Source: CAD feature listing. Evaluate the final solid. Frame: model axes, mm. Face numbers are marked on the shaded views. A direction names the side the tool comes from. Give positions to 0.01 mm unless a question says otherwise; leave off trailing zeros. Order: outer loops, then holes, each group sorted by start corner. A loop starts at its lowest first (then second) coordinate and runs counter-clockwise, first axis right, second up. Notation, with made-up numbers: (-4.75, -4.75) -> (21.25, -4.75) arc R29 ccw to (21.25, 32.25) -> close; hole circle Ø8 at (33.5, 10). An arc over 180 degrees is marked (long way). Answer in a Markdown table with one row per item.
Autodesk Inventor part; units mm, degrees
ref_plane "YZ Plane" through (0, 0, 0) normal (1, 0, 0) x (0, 1, 0)
ref_plane "XZ Plane" through (0, 0, 0) normal (0, 1, 0) x (-1, 0, 0)
ref_plane "XY Plane" through (0, 0, 0) normal (0, 0, 1) x (1, 0, 0)
sketch "Sketch1" plane through (0, 0, 0) normal (0, 0, 1) x (1, 0, 0)
  line L0 (0, 34.8483) -> (20, 34.8483)
  line L1 (20, 34.8483) -> (20, 29.9983)
  line L2 (0, 34.8483) -> (0, 0)
  line L3 (20, 29.9983) -> (5, 29.9983)
  line L4 (5, 29.9983) -> (5, 7.1983)
  line L5 (5, 7.1983) -> (20, 7.1983)
  line L6 (20, 7.1983) -> (20, 2.3483)
  line L7 (20, 2.3483) -> (5, 2.3483)
  line L8 (0, 0) -> (0, -15.1517)
  line L9 (5, -15.1517) -> (5, 2.3483)
  line L10 (5, -15.1517) -> (5, -22.2152)
  arc A0 (0, -15.1517) -> (5, -22.2152) centre (9.8436, -13.4852) ccw
  dimension "d14" = 20
  dimension "d15" = 4.85
  dimension "d17" = 4.85
  dimension "d18" = 22.8
  dimension "d19" = 20
  dimension "d20" = 5
  dimension "d22" = 9.9837
  dimension "d23" = 90
  dimension "d24" = 29.9983
  dimension "d25" = 10.1564
  dimension "d26" = 43.4835
  dimension "d27" = 45.15
extrude "Extrusion1" add sketch "Sketch1" against normal blind 10
sketch "Sketch2" plane through (20, 29.9983, 0) normal (1, 0, 0) x (0, 0, -1)
  line L0 (0, 0) -> (10, 0)
  line L1 (2, 0) -> (2, 4.85)
  line L2 (0, 4.85) -> (10, 4.85)
  line L3 (2, 4.85) -> (10, 4.85)
  line L4 (10, 4.85) -> (10, 0)
  line L5 (10, -45.15) -> (10, 4.85)
  line L6 (0, 0) -> (0, 4.85)
  line L7 (0, 0) -> (10, 0)
  line L8 (2, 0) -> (10, 0)
  line L9 (10, -22.8) -> (10, -27.65)
  line L10 (2, -27.65) -> (2, -22.8)
  line L11 (2, -22.8) -> (10, -22.8)
  line L12 (10, -22.8) -> (10, -27.65)
  line L13 (2, -27.65) -> (10, -27.65)
  point P0 (0, -29.9983)
  point P1 (10, -11.4)
  dimension "d30" = 2
  dimension "d33" = 11.4
  dimension "d36" = 27.65
extrude "Extrusion2" cut sketch "Sketch2" against normal blind 15 contours L5 L13 L10 L11 | L1 L2 L4 L0
fillet "Fillet1" radius 1 1 edges at (5, -22.2152, -5)
sketch "Sketch3" plane through (0, 0, 0) normal (0, 0, 1) x (1, 0, 0)
  line L0 (20, 34.8483) -> (0, 34.8483)
  line L1 (5, 7.1983) -> (5, 29.9983)
  circle A0 centre (11.05, 32.4233) radius 1.1
  circle A1 centre (11.05, 4.7733) radius 1.1
  point P0 (0, 0)
  dimension "d42" = 2.425
  dimension "d43" = 6.05
  dimension "d44" = 1.1
  dimension "d47" = 27.65
extrude "Extrusion3" cut sketch "Sketch3" against normal blind 15
properties part number "first joint"
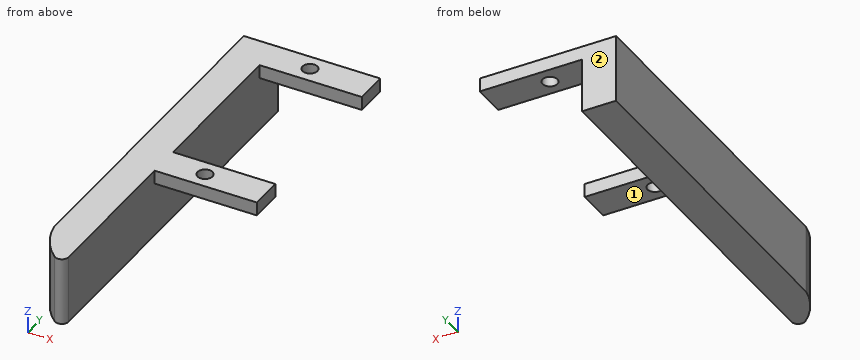
(1) First-contact query: pin 1 Ø5.5 at (x, y) = (9.5, 4.5) entering from -Z; pin 2 Ø1.6 at (x, z) = (15, -1) entering from -Y; pin 3 Ø3 at (x, z) = (12.5, -5) entering from -Y. Flat tips, straight axial feed; report the tip coordinate or a pass-through.
A:
| item | result |
|---|---|
| pin 1 | stops at z = -2 |
| pin 2 | stops at y = 2.35 |
| pin 3 | passes through |
(2) Section query D-D (y = -13). Return the cut outline in (x, z).
A:
| item | result |
|---|---|
| outline | (0, -10) -> (5, -10) -> (5, 0) -> (0, 0) -> close |
(3) Section query C-C (z = -1.5). Return the cut outline in (x, y), plus the area to 3 significant figures.
A:
| item | result |
|---|---|
| outline | (0, -15.15) arc R9.98 ccw to (3.35, -21.07) arc R1 ccw to (5, -20.31) -> (5, 2.35) -> (20, 2.35) -> (20, 7.2) -> (5, 7.2) -> (5, 30) -> (20, 30) -> (20, 34.85) -> (0, 34.85) -> close; hole circle Ø2.2 at (11.05, 4.77); hole circle Ø2.2 at (11.05, 32.42) |
| area | 410 mm^2 |
(4) Ray query, probe 1 along Y at (x, z) = (11.05, -0.65); probe 2 along Y at (x, z) = (17.75, -1); probe 3 along Z at (x, y) = (19, 6). Return the intervals inside material, ascending.
A:
| item | result |
|---|---|
| probe 1 | y = 2.35 to 3.67, 5.87 to 7.2, 30 to 31.32, 33.52 to 34.85 |
| probe 2 | y = 2.35 to 7.2, 30 to 34.85 |
| probe 3 | z = -2 to 0 |
(5) Section query B-B (x = 11.05). Return the cut outline in (y, z).
A:
| item | result |
|---|---|
| outline | (2.35, -2) -> (3.67, -2) -> (3.67, 0) -> (2.35, 0) -> close; (5.87, -2) -> (7.2, -2) -> (7.2, 0) -> (5.87, 0) -> close; (30, -2) -> (31.32, -2) -> (31.32, 0) -> (30, 0) -> close; (33.52, -2) -> (34.85, -2) -> (34.85, 0) -> (33.52, 0) -> close |
(6) Access query for the marked faces 1 and 2. Directions: +Z, -Z, +X, -X, +Y, -Y. A direction counts if a zero-diameter tool reaches every point of the face in a straight line with its end or side. Return the directions, or none.
A:
| item | result |
|---|---|
| face 1 | -Z, +X, +Y, -Y |
| face 2 | +Z, -Z, +X, -X, +Y |
(7) Section query A-A (x = 5.5). Return the cut outline in (y, z), plus the area to 3 significant figures.
A:
| item | result |
|---|---|
| outline | (2.35, -2) -> (7.2, -2) -> (7.2, 0) -> (2.35, 0) -> close; (30, -2) -> (34.85, -2) -> (34.85, 0) -> (30, 0) -> close |
| area | 19.4 mm^2 |
